Design review of the part built by this model. Coordinates are the model's own, in mm. Coordinates: 2 decimals unless noted, no trailing zeros. Write each loop counter-clockwise with the first axis right and the second up, starting at its lowest first coordinate (ties: lowest second). Pieces come first, ordered by that corner, then holes. Notation, with made-up numbers: M 2,60 L 17,60 A16 ccw 17,76 Z; hole C -10.5,2.25 d5. An arc over 180 degrees is marked long. Write each question's results on one line, items separated by ' | '. Start each with the question number.
```python
from build123d import *

# Parameters (mm, degrees)
F0_R     = 50.8
F1_DEPTH = 9.525
F2_R     = 15.875
F3_DEPTH = 9.526
F5_D     = 6.6
F6_R     = 3.3
F7_DEPTH = 9.526


with BuildPart() as f1:
    # F0 (on Top) → F1 (new body)
    with BuildSketch(Plane.XY):
        Circle(F0_R)
    extrude(amount=F1_DEPTH)

    # F2 (on face) → F3 (cut, through all)
    with BuildSketch(Plane.XY.offset(9.525)):
        Circle(F2_R)
    extrude(amount=-F3_DEPTH, mode=Mode.SUBTRACT)

    # F5 (through all)
    with Locations(Plane.XY.offset(9.525)):
        with Locations((-13.3652133, 32.2664949823), (-32.2664903636, 13.3652244507), (-32.2664949823, -13.3652133), (-13.3652244507, -32.2664903636), (13.3652133, -32.2664949823), (32.2664903636, -13.3652244507), (32.2664949823, 13.3652133), (13.3652244507, 32.2664903636)):
            Hole(F5_D / 2)

    # F6 (on face) → F7 (cut, through all)
    with BuildSketch(Plane.XY.offset(9.525)):
        with BuildLine():
            Line((92.0014753938, 88.4870588779), (0, 88.4870588779))
            Line((0, 88.4870588779), (0, 50.8))
            ThreePointArc((0, 50.8), (35.9210244843, 35.9210244843), (50.8, 0))
            ThreePointArc((50.8, 0), (35.9210244843, -35.9210244843), (0, -50.8))
            Line((0, -50.8), (0, -93.3939293027))
            Line((0, -93.3939293027), (92.0014753938, -93.3939293027))
            Line((92.0014753938, -93.3939293027), (92.0014753938, 88.4870588779))
        make_face()
        with BuildLine():
            ThreePointArc((50.8, 0), (35.9210244843, 35.9210244843), (0, 50.8))
            Line((0, 50.8), (0, 15.875))
            ThreePointArc((0, 15.875), (11.2253201513, 11.2253201513), (15.875, 0))
            ThreePointArc((15.875, 0), (11.2253201513, -11.2253201513), (0, -15.875))
            Line((0, -15.875), (0, -50.8))
            ThreePointArc((0, -50.8), (35.9210244843, -35.9210244843), (50.8, 0))
        make_face()
        with Locations((13.3652133, -32.2664949823)):
            Circle(F6_R, mode=Mode.SUBTRACT)
        with Locations((32.2664903636, -13.3652244507)):
            Circle(F6_R, mode=Mode.SUBTRACT)
        with Locations((13.3652244507, 32.2664903636)):
            Circle(F6_R, mode=Mode.SUBTRACT)
        with Locations((32.2664949823, 13.3652133)):
            Circle(F6_R, mode=Mode.SUBTRACT)
    extrude(amount=-F7_DEPTH, mode=Mode.SUBTRACT)


solid = f1.part
```
Item 1: Draft analysis for pull direction X (two halves, no side actions). For faces 1 (the cylindrical face through (-15.87, 0.35, 4.83)), 2 (the cylindrical face through (-35.315, -14.629, 4.696)), 3 (the flat face through (-26, 1, 0)), 4 (the cylindrical face through (-12.9, -29, 4.7)), state which applies: released by +X, released by -X, zero draft, split by the parting line, or undercut.
Item 2: We need section C-C on y = 0. State the section outline as (x, z) points (3 decimals).
Item 3: We need section A-A on x = -8.5. State the section outline as (y, z) points (3 decimals), then the cut area to 3 significant figures.
Item 4: We need section B-B on z = 2. Count the separate pieces of the cut face and the enclosed holes in it, then the cut area to 3 significant figures.
Item 5: We need section D-D on x = -41.5. State the section outline as (y, z) points (3 decimals).
Item 6: Insertion check: pin 1 Ø7.5 at (x, y) = (-32.27, -13.37) entering from +Z (3 decimals); pin 2 Ø2 at (y, z) = (-34, 2) entering from -X; pin 3 Ø2 at (x, z) = (-45, 4) entering from +Y; pin 4 Ø5.5 at (x, y) = (-13.37, -32.27) entering from -Z. Each pin has a flat end and moves straight along its axis. Give the tip position at first contact, or say it passes through.
Item 7: Wall thickness on L1, parallel to Y at x = -11.5, z = 4.5; L2, parallel to Y at x = -11, z = 2.5; L3, parallel to Y at x = -16, z = 7: over which ranges is each line inside the solid? List them lowest first.
Answer:
1) face 1: released by +X | face 2: undercut | face 3: zero draft | face 4: undercut
2) outline: M -50.8,0 L -15.875,0 L -15.875,9.525 L -50.8,9.525 Z
3) outline: M -50.084,0 L -13.408,0 L -13.408,9.525 L -50.084,9.525 Z; M 13.408,0 L 50.084,0 L 50.084,9.525 L 13.408,9.525 Z | area: 699 mm^2
4) separate pieces: 1 | enclosed holes: 4 | area: 3,520 mm^2
5) outline: M -29.298,0 L 29.298,0 L 29.298,9.525 L -29.298,9.525 Z
6) pin 1: stops at z = 9.525 | pin 2: stops at x = -38.62 | pin 3: stops at y = 25.39 | pin 4: passes through
7) L1: y = -49.48 to -34.99, -29.54 to -10.94, 10.94 to 29.54, 34.99 to 49.48 | L2: y = -49.59 to -34.57, -29.97 to -11.45, 11.45 to 29.97, 34.57 to 49.59 | L3: y = -48.21 to -34.25, -30.28 to 30.28, 34.25 to 48.21
